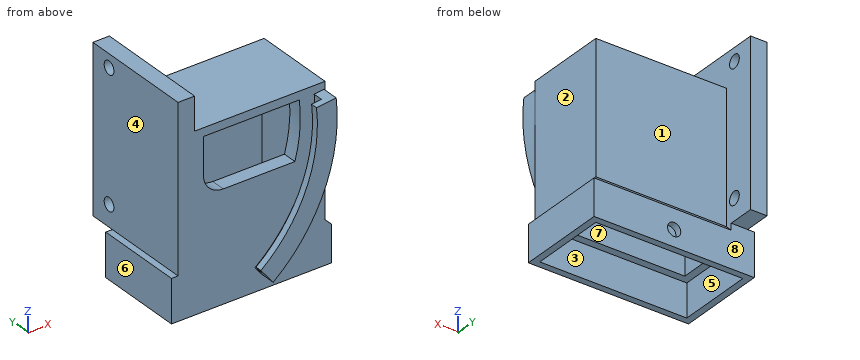
from build123d import *

# Parameters (mm, degrees)
SKETCH1_W                = 44.5
SKETCH1_H                = 25.05
SKETCH1_W_2              = 39.9
SKETCH1_H_2              = 18.45
BOSS_EXTRUDE1_DEPTH      = 40
BOSS_EXTRUDE2_START      = 40
BOSS_EXTRUDE2_OUTLINE_W  = 44.5
BOSS_EXTRUDE2_OUTLINE_H  = 25.05
BOSS_EXTRUDE2_DEPTH      = 2.5
BOSS_EXTRUDE3_DEPTH      = 3
BOSS_EXTRUDE3_DEPTH_BACK = 10
SKETCH1_4_W              = 48.5
SKETCH1_4_H              = 27.05
SKETCH1_4_W_2            = 44.5
SKETCH1_4_H_2            = 23.05
SKETCH2_W                = 5
SKETCH2_H                = 25.05
BOSS_EXTRUDE4_DEPTH      = 10
CUT_EXTRUDE1_REACH       = 65.844
SKETCH7_W                = 5
SKETCH7_H                = 49.5
BOSS_EXTRUDE5_DEPTH      = 10
SKETCH8_R                = 2
CUT_EXTRUDE2_DEPTH       = 5.8
CHAMFER1_SIZE            = 2
CHAMFER2_SIZE            = 2
SKETCH9_R                = 2
CUT_EXTRUDE3_DEPTH       = 10


# Read off the part's stored shape, not the designer's step: Boss-Extrude2
with BuildPart() as part:
    # Sketch1 → Boss-Extrude1 (new body)
    with BuildSketch(Plane.XY):
        with Locations((0, -1)):
            Rectangle(SKETCH1_W, SKETCH1_H)
        Rectangle(SKETCH1_W_2, SKETCH1_H_2, mode=Mode.SUBTRACT)
    extrude(amount=BOSS_EXTRUDE1_DEPTH)

    # Boss-Extrude2 outline → Boss-Extrude2 (add)
    with BuildSketch(Plane.XY.offset(BOSS_EXTRUDE2_START)):
        with Locations((0, -1)):
            Rectangle(BOSS_EXTRUDE2_OUTLINE_W, BOSS_EXTRUDE2_OUTLINE_H)
    extrude(amount=BOSS_EXTRUDE2_DEPTH)

    # Sketch1<4> → Boss-Extrude3 (add, two sides: drawn at the far end of the back side and taken through both)
    with BuildSketch(Plane.XY.offset(-BOSS_EXTRUDE3_DEPTH_BACK)):
        Rectangle(SKETCH1_4_W, SKETCH1_4_H)
        Rectangle(SKETCH1_4_W_2, SKETCH1_4_H_2, mode=Mode.SUBTRACT)
    extrude(amount=BOSS_EXTRUDE3_DEPTH + BOSS_EXTRUDE3_DEPTH_BACK)

    # Sketch2 → Boss-Extrude4 (add)
    with BuildSketch(Plane.XY.offset(42.5)):
        with Locations((-19.75, -1)):
            Rectangle(SKETCH2_W, SKETCH2_H)
    extrude(amount=BOSS_EXTRUDE4_DEPTH)

    # Sweep1: sweep along a path in Sketch4
    with BuildLine(Plane.XZ.offset(13.525)) as sweep1_path:
        ThreePointArc((1.009931304, -3.080074503), (15.529238499, 16.150172823), (18.964123835, 40))
    # Sketch6 → Sweep1 (sweep)
    with BuildSketch(Plane(origin=(18.964123835, -13.525, 40), x_dir=(0.9940873595600267, 0, 0.10858324715615325), z_dir=(-0.10858324715615325, 0, 0.9940873595600267))):
        Polygon((-0.007155114, -3), (-3.007155114, -3), (-3.007155114, -5), (2.992844886, -5), (2.992844886, -1.848135777), (2.992844886, 0), (-0.007155114, 0), align=None)
    sweep(path=sweep1_path.line)

    # Sketch4<3> → Cut-Extrude1 (cut, up to next)
    with BuildSketch(Plane.XZ.offset(13.525), mode=Mode.PRIVATE) as cut_extrude1_sk1:
        with BuildLine():
            Line((-14.565566912, 40), (14.442409674, 40))
            ThreePointArc((14.442409674, 40), (14.628132166, 31.380371303), (13.124010953, 22.890959598))
            Line((13.124010953, 22.890959598), (-8.565566912, 22.890959598))
            ThreePointArc((-8.565566912, 22.890959598), (-12.808207599, 24.648318911), (-14.565566912, 28.890959598))
            Line((-14.565566912, 28.890959598), (-14.565566912, 40))
        make_face()
    cut_extrude1_tool1 = extrude(cut_extrude1_sk1.sketch, amount=-CUT_EXTRUDE1_REACH, mode=Mode.PRIVATE) & part.part
    add(cut_extrude1_tool1.solids().sort_by_distance((0.104414, -13.525, 31.62544))[0], mode=Mode.SUBTRACT)

    # Sketch7 → Boss-Extrude5 (add)
    with BuildSketch(Plane(origin=(0, 11.525, 0), x_dir=(1, 0, 0), z_dir=(0, 1, 0))):
        with Locations((-19.75, -27.75)):
            Rectangle(SKETCH7_W, SKETCH7_H)
    extrude(amount=BOSS_EXTRUDE5_DEPTH)

    # Sketch8 → Cut-Extrude2 (cut)
    with BuildSketch(Plane.ZY.offset(22.25)):
        with Locations(Location((48.5, 14.875, 0), (0, 0, 270))):
            Circle(SKETCH8_R)
        with Locations(Location((9.5, 14.875, 0), (0, 0, 270))):
            Circle(SKETCH8_R)
    extrude(amount=-CUT_EXTRUDE2_DEPTH, mode=Mode.SUBTRACT)

    # Chamfer1
    chamfer1_edges = [part.edges().sort_by_distance(p)[0] for p in [
        (3.5, 13.525, 3),
    ]]
    chamfer(chamfer1_edges, length=CHAMFER1_SIZE - 0.0001)  # a hair under: the kernel refuses the full size

    # Chamfer2
    chamfer2_edges = [part.edges().sort_by_distance(p)[0] for p in [
        (24.25, -0.99995, 3),
    ]]
    chamfer(chamfer2_edges, length=CHAMFER2_SIZE)

    # Sketch9 → Cut-Extrude3 (cut)
    with BuildSketch(Plane(origin=(0, 13.525, 0), x_dir=(1, 0, 0), z_dir=(0, 1, 0))):
        with Locations(Location((0, 5, 0), (0, 0, 180))):
            Circle(SKETCH9_R)
    extrude(amount=-CUT_EXTRUDE3_DEPTH, mode=Mode.SUBTRACT)


solid = part.part
Source: CAD feature listing. Evaluate the final solid. Frame: model axes, mm. Face numbers are marked on the shaded views. A direction names the side the tool comes from. Round coordinates to 2 decimals unless told otherwise and drop trailing zeros. Write each loop counter-clockwise with the first axis right and the second up, starting at its lowest first coordinate (ties: lowest second). Pieces come first, ordered by that corner, then holes. Notation, with made-up numbers: (64, 57) - (119, 57) arc R10 ccw to (119, 65) - close; hole circle Ø6 at (32.25, 22.5). An arc over 180 degrees is marked (long way). Use CSV: the item, a comma, the result in double quotes. Start each with the question number.
(1) Mould query, pull axis Y, two halves, no side actions, for the marked faces 5, 6, 7 and 8. Classes: pulls with the +Y half, pulls with the -Y half, needs draft (parallel to the pull), parting line crosses it, or undercut.
(2) Cut plane D-D, the plane z = 48.5. Return loops of the section in (x, y) (3 decimals), and give its area (3 significant figures).
(3) Cut plane A-A, the plane z = 9.5. Return loops of the section in (x, y) (3 decimals).
(4) Set-up query: the marked faces 1, 2, 3 and 4. Return all of +Z, -Z, +X, -X, +Y, -Y with unobstructed straight access to the full face (end or side cutting, diameter ignored); none if empty.
(5) Cut plane B-B, the plane x = -18.5. Return loops of the section in (y, z) (3 decimals).
(6) Material intervals for probe 1 along Y at (x, z) = (9, 3) (3 decimals); probe 2 along Z at (x, y) = (0, -13); probe 3 along X at (y, z) = (-8.5, 26.5), sorted ascending. Write a range as [from, to].
(7) First-contact query: pin 1 Ø3 at (x, y) = (10.5, 3.5) entering from -Z; pin 2 Ø8 at (x, z) = (-2, -4) entering from -Y (3 decimals); pin 3 Ø6 at (x, z) = (11, 22) entering from +Y (3 decimals); pin 4 Ø9 at (y, z) = (2.5, 10.5) entering from -X. Flat tips, straight axial feed; report the tip coordinate or a pass-through.
(8) Cut plane C-C, the plane y = -1. Return loops of the section in (x, z).
Geometry says:
1,face 5,"undercut"
1,face 6,"needs draft"
1,face 7,"undercut"
1,face 8,"pulls with the +Y half"
2,outline,"(-22.25, -13.525) - (-17.25, -13.525) - (-17.25, 12.875) - (-22.25, 12.875) - close; (-22.25, 16.875) - (-17.25, 16.875) - (-17.25, 21.525) - (-22.25, 21.525) - close"
2,area,"155 mm²"
3,outline,"(-22.25, -13.525) - (12.125, -13.525) - (12.125, -16.525) - (8.562, -16.525) - (8.562, -18.525) - (15.605, -18.525) - (15.605, -13.525) - (22.25, -13.525) - (22.25, 11.525) - (-17.25, 11.525) - (-17.25, 12.875) - (-22.25, 12.875) - close; (-22.25, 16.875) - (-17.25, 16.875) - (-17.25, 21.525) - (-22.25, 21.525) - close; hole (-19.95, -9.225) - (19.95, -9.225) - (19.95, 9.225) - (-19.95, 9.225) - close"
4,face 1,"+Z, +X, +Y"
4,face 2,"+Z, +X, +Y, -Y"
4,face 3,"-Z"
4,face 4,"+Z, -X, +Y, -Y"
5,outline,"(-13.525, -10) - (-11.525, -10) - (-11.525, 0) - (-9.225, 0) - (-9.225, 40) - (9.225, 40) - (9.225, 0) - (11.525, 0) - (11.525, -10) - (13.525, -10) - (13.525, 3) - (21.525, 3) - (21.525, 52.5) - (-13.525, 52.5) - close; hole circle Ø4 at (14.875, 9.5); hole circle Ø4 at (14.875, 48.5)"
6,probe 1,"[-18.525, -9.225], [9.225, 11.525]"
6,probe 2,"[-10, 22.89], [40, 42.5]"
6,probe 3,"[-22.25, -19.95], [19.95, 22.25]"
7,pin 1,"z = 40"
7,pin 2,"y = -18.525"
7,pin 3,"y = 11.525"
7,pin 4,"x = -22.25"
8,outline,"(-24.25, -10) - (-22.25, -10) - (-22.25, 0) - (-19.95, 0) - (-19.95, 40) - (19.95, 40) - (19.95, 0) - (22.25, 0) - (22.25, -10) - (24.25, -10) - (24.25, 1) - (22.25, 3) - (22.25, 42.5) - (-17.25, 42.5) - (-17.25, 52.5) - (-22.25, 52.5) - (-22.25, 3) - (-24.25, 3) - close"
